from build123d import *

# Parameters (mm, degrees)
PROFILE_SKETCH_R              = 10
PROFILE_SKETCH_R_2            = 5
CYLINDER_EXTRUDE_DEPTH        = 9
LIP_RING_SKETCH_R             = 7
LIP_RING_SKETCH_R_2           = 5
BOTTOM_LIP_RING_EXTRUDE_DEPTH = 1
BOTTOM_RING_FILLET_R          = 1
TOP_START                     = -10
SKETCH2_2_R                   = 7
SKETCH2_2_R_2                 = 5
TOP_LIP_RING_EXTRUDE_DEPTH    = 1
TOP_RING_FILLET_R             = 1


with BuildPart() as part:
    # Profile Sketch → Cylinder Extrude (new body)
    with BuildSketch(Plane(origin=(0, 0, 0), x_dir=(1, 0, 0), z_dir=(0, 1, 0))):
        with Locations(Location((0, 0, 0), (0, 0, 270))):
            Circle(PROFILE_SKETCH_R)
        with Locations(Location((0, 0, 0), (0, 0, 270))):
            Circle(PROFILE_SKETCH_R_2, mode=Mode.SUBTRACT)
    extrude(amount=CYLINDER_EXTRUDE_DEPTH)

    # Lip Ring Sketch → Bottom Lip Ring Extrude (add)
    with BuildSketch(Plane(origin=(0, 9, 0), x_dir=(1, 0, 0), z_dir=(0, 1, 0))):
        with Locations(Location((0, 0, 0), (0, 0, 270))):
            Circle(LIP_RING_SKETCH_R)
        with Locations(Location((0, 0, 0), (0, 0, 270))):
            Circle(LIP_RING_SKETCH_R_2, mode=Mode.SUBTRACT)
    extrude(amount=BOTTOM_LIP_RING_EXTRUDE_DEPTH)

    # Bottom Ring Fillet
    bottom_ring_fillet_edges = [part.edges().sort_by_distance(p)[0] for p in [
        (0, 10, -7),
        (0, 10, -5),
    ]]
    fillet(bottom_ring_fillet_edges, radius=BOTTOM_RING_FILLET_R - 0.0001)  # a hair under: the kernel refuses the full size

    # Sketch2<2> → Top Lip Ring Extrude (add)
    with BuildSketch(Plane(origin=(0, 9, 0), x_dir=(1, 0, 0), z_dir=(0, 1, 0)).offset(TOP_START)):
        with Locations(Location((0, 0, 0), (0, 0, 270))):
            Circle(SKETCH2_2_R)
        with Locations(Location((0, 0, 0), (0, 0, 270))):
            Circle(SKETCH2_2_R_2, mode=Mode.SUBTRACT)
    extrude(amount=TOP_LIP_RING_EXTRUDE_DEPTH)

    # Top Ring Fillet
    top_ring_fillet_edges = [part.edges().sort_by_distance(p)[0] for p in [
        (0, -1, -7),
        (0, -1, -5),
    ]]
    fillet(top_ring_fillet_edges, radius=TOP_RING_FILLET_R - 0.0001)  # a hair under: the kernel refuses the full size


solid = part.part
The listing builds one solid part. Answer for the finished solid, in the listing's coordinates (mm). Give positions to 0.01 mm unless a question says otherwise; leave off trailing zeros. Loops run counter-clockwise (first coordinate to the right, second up) from the corner with the lowest first, then second, coordinate; pieces in that order, holes last. Notation, with made-up numbers: (81.5, 21.5) - (86.5, 21.5) arc R12 ccw to (86.5, 31.5) - close; hole circle Ø5 at (7.5, -29.75). An arc over 180 degrees is marked (long way). Write each question's results on one line, items separated by ' | '.
1. Consider probe 1 along X at (y, z) = (4, 0); probe 2 along X at (y, z) = (3.5, -1.75); probe 3 along Y at (x, z) = (-5.5, -5). Determine where each line is inside the solid, lowest interval first. Write a range as from..to.
Resolved:
probe 1: x = -10..-5, 5..10 | probe 2: x = -9.85..-4.68, 4.68..9.85 | probe 3: y = 0..9
2. For a pull along Z with two mould halves and no side action, classify faces 1 (the face through (-9.76, 4.44, -2.17)), 2 (the face through (7, 9, 2)), 3 (the face through (-4.88, 4.44, -1.08)) as +Z half, -Z half, draft (parallel to the pull), parting line (faces both ways), or undercut.
Resolved:
face 1: parting line | face 2: draft | face 3: undercut
3. Flat-ended cylindrical pins translate along their axes: P1, Ø1.5, axis at y = 2, z = -2, coming from the +X side; P2, Ø2, axis at x = -1.5, z = 4.5, coming from the +Y side; P3, Ø1, axis at y = 2, z = 6.5, coming from the -X side. Find the tip coordinate at first contact, or state that the pin passes through.
Resolved:
P1: stops at x = 9.92 | P2: stops at y = 9.97 | P3: stops at x = -8
4. Find section D-D, the plane x = -8.25. Write down the section's boundary in (y, z).
Resolved:
outline: (0, -5.65) - (9, -5.65) - (9, 5.65) - (0, 5.65) - close
5. Find section C-C, the plane y = 1.25. Write down the section's boundary in (x, z).
Resolved:
outline: circle Ø20 at (0, 0); hole circle Ø10 at (0, 0)
